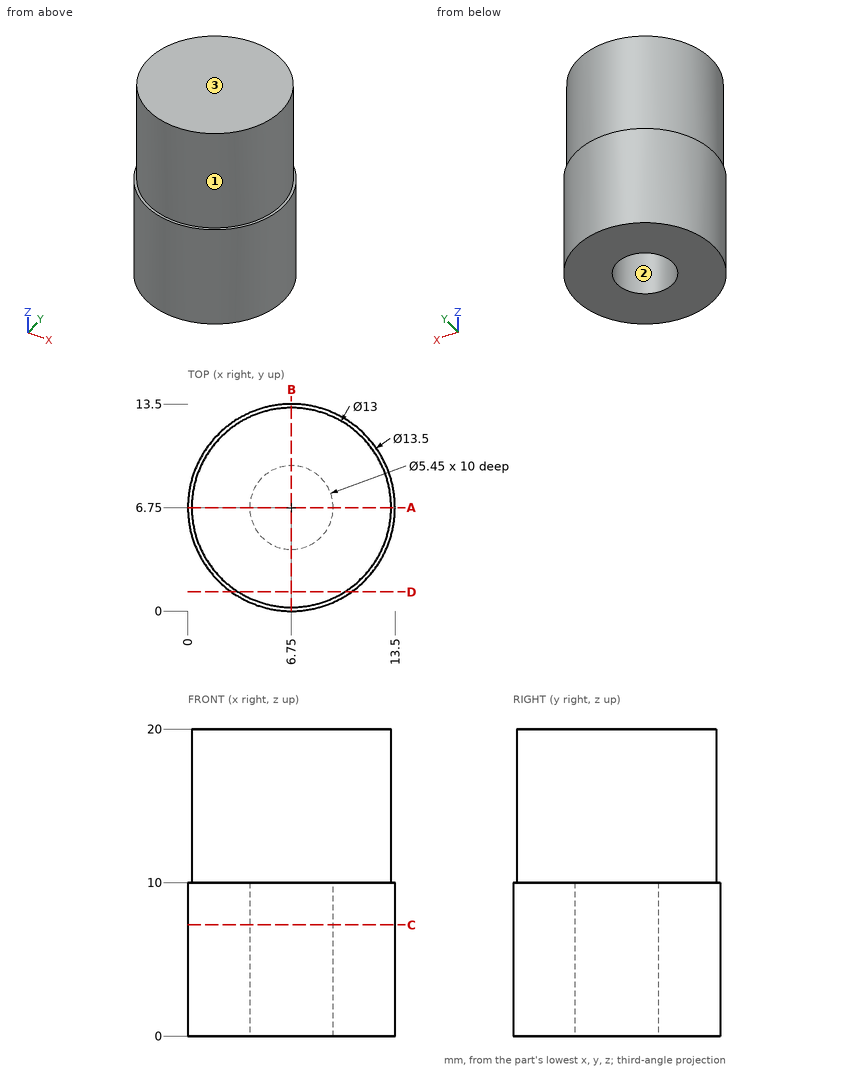
Could you check a few things on this drawing? It's one solid part, dimensions in mm from its lowest x, y, z. A direction names the side the tool comes from. Coordinates: 2 decimals unless noted, no trailing zeros. Order: outer loops, then holes, each group sorted by start corner. A loop starts at its lowest first (then second) coordinate and runs counter-clockwise, first axis right, second up. Notation, with made-up numbers: (62.5, 68) - (93.5, 68) arc R22 cw to (93.5, 90) - close; hole circle Ø10 at (43.25, -7.5). An arc over 180 degrees is marked (long way). One line per question, with ' | ' between items. Start each with the question number.
1. I'm going to push flat-ended pins straight in: pin 1 Ø4 at (x, z) = (6, 4.5) entering from +Y; pin 2 Ø1.5 at (x, z) = (3, 3) entering from +Y; pin 3 Ø5 at (x, z) = (12, 17) entering from +Y; pin 4 Ø2 at (y, z) = (3.5, 11.5) entering from +X. Where does each tip first touch, or does it pass through?
2. Please list where these lines run through material, in increasing order: line 1 along Y through (x, z) = (6.75, 4.75) (3 decimals); line 2 along X through (y, z) = (4.5, 6.75); line 3 along Y through (x, z) = (9.25, 8). Write a range as [from, to].
3. Which directions (+Z, -Z, +X, -X, +Y, -Y) give clear straight access to the entire face, cutting with the end or side of a thin tool? Please do the marked faces 1, 2 and 3.
4. If we section it at A-A (y = 6.75): Write out the boundary of the cut face in (x, z) (3 decimals), and give its area (4 significant figures).
5. If we section it at C-C (z = 7.25): Write out the boundary of the cut face in (x, y) (3 decimals), and give its area (3 significant figures).
6. If we section it at D-D (y = 1.25): Write out the boundary of the cut face in (x, z).
Model answer:
1) pin 1: stops at y = 13.5 | pin 2: stops at y = 12.8 | pin 3: stops at y = 12.64 | pin 4: stops at x = 12.85
2) line 1: y = [0, 4.025], [9.475, 13.5] | line 2: x = [0.39, 5.21], [8.29, 13.11] | line 3: y = [0.48, 5.67], [7.83, 13.02]
3) face 1: +Z | face 2: -Z | face 3: +Z, +X, -X, +Y, -Y
4) outline: (0, 0) - (4.025, 0) - (4.025, 10) - (9.475, 10) - (9.475, 0) - (13.5, 0) - (13.5, 10) - (13.25, 10) - (13.25, 20) - (0.25, 20) - (0.25, 10) - (0, 10) - close | area: 210.5 mm²
5) outline: circle Ø13.5 at (6.75, 6.75); hole circle Ø5.45 at (6.75, 6.75) | area: 120 mm²
6) outline: (2.84, 0) - (10.66, 0) - (10.66, 10) - (10.21, 10) - (10.21, 20) - (3.29, 20) - (3.29, 10) - (2.84, 10) - close
